The listing builds one solid part. Answer for the finished solid, in the listing's coordinates (mm). A direction names the side the tool comes from. Round coordinates to 2 decimals unless told otherwise and drop trailing zeros. Loops run counter-clockwise (first coordinate to the right, second up) from the corner with the lowest first, then second, coordinate; pieces in that order, holes last. Notation, with made-up numbers: (-25, 1.25) -> (12, 1.25) arc R23 ccw to (12, 30.25) -> close; hole circle Ø4 at (73, -31). An arc over 180 degrees is marked (long way). Use a Markdown table: item, result. Add a question column.
Q1. Section A-A on x = 0 is taken. Give the vertices of the cut face in (y, z).
Q2. Section B-B on z = -5 is taken. Give the vertices of the cut face in (x, y).
Q3. Which of the six approach directions +Z, -Z, +X, -X, +Y, -Y give full straight-line access (tool end or side, diameter ignored) to faces 1 (the flat face through (-1.4, 0, -4.5)), 2 (the cylindrical face through (-6, 31, 0))?
Q4. Consider line 1 (Y direction, x = -1.75, z = 5.5); line 2 (X direction, y = 19.5, z = 0.25); line 3 (X direction, y = 26.5, z = 2.5). Determine where each line is inside the solid, lowest interval first.
Q5. Section C-C on y = 22.5 is taken. Give the vertices of the cut face in (x, z), then the cut area to 3 significant figures.
Q6. Section D-D on z = 0 is taken. Give the vertices of the cut face in (x, y).
Q7. For a pull along Y with two mould halves and no side action, classify faces 3 (the cylindrical face through (-0.59, 14.79, -4.46)), 4 (the flat face through (0, -2, 0)), 5 (the cylindrical face through (-6, -1, 0)) as released by +Y, released by -Y, zero draft, split by the parting line, or undercut.
Q8. Given pin 1 Ø5 at (x, y) = (-4.5, 6.5) entering from +Z; pin 2 Ø1.5 at (y, z) = (26, 2) entering from -X; pin 3 Ø1 at (x, y) = (2, 2.5) entering from -Z, each flat-ended and moving along its own axis, determine where each tip first touches the part or whether it passes through.
from build123d import *

# Parameters (mm, degrees)
SKETCH1_R           = 4.5
BOSS_EXTRUDE1_DEPTH = 30
SKETCH2_R           = 6
BOSS_EXTRUDE2_DEPTH = 2
SKETCH3_R           = 6
BOSS_EXTRUDE3_DEPTH = 2


with BuildPart() as part:
    # Sketch1 → Boss-Extrude1 (new body)
    with BuildSketch(Plane(origin=(0, 0, 0), x_dir=(1, 0, 0), z_dir=(0, 1, 0))):
        Circle(SKETCH1_R)
    extrude(amount=BOSS_EXTRUDE1_DEPTH)

    # Sketch2 → Boss-Extrude2 (add)
    with BuildSketch(Plane(origin=(0, 0, 0), x_dir=(1, 0, 0), z_dir=(0, 1, 0))):
        Circle(SKETCH2_R)
    extrude(amount=-BOSS_EXTRUDE2_DEPTH)

    # Sketch3 → Boss-Extrude3 (add)
    with BuildSketch(Plane(origin=(0, 30, 0), x_dir=(1, 0, 0), z_dir=(0, 1, 0))):
        Circle(SKETCH3_R)
    extrude(amount=BOSS_EXTRUDE3_DEPTH)


solid = part.part
Checked values:
| question | item | result |
|---|---|---|
| 1 | outline | (-2, -6) -> (0, -6) -> (0, -4.5) -> (30, -4.5) -> (30, -6) -> (32, -6) -> (32, 6) -> (30, 6) -> (30, 4.5) -> (0, 4.5) -> (0, 6) -> (-2, 6) -> close |
| 2 | outline | (-3.32, -2) -> (3.32, -2) -> (3.32, 0) -> (-3.32, 0) -> close; (-3.32, 30) -> (3.32, 30) -> (3.32, 32) -> (-3.32, 32) -> close |
| 3 | face 1 | none |
| 3 | face 2 | +Y, -Y |
| 4 | line 1 | y = -2 to 0, 30 to 32 |
| 4 | line 2 | x = -4.49 to 4.49 |
| 4 | line 3 | x = -3.74 to 3.74 |
| 5 | outline | circle Ø9 at (0, 0) |
| 5 | area | 63.6 mm2 |
| 6 | outline | (-6, -2) -> (6, -2) -> (6, 0) -> (4.5, 0) -> (4.5, 30) -> (6, 30) -> (6, 32) -> (-6, 32) -> (-6, 30) -> (-4.5, 30) -> (-4.5, 0) -> (-6, 0) -> close |
| 7 | face 3 | undercut |
| 7 | face 4 | released by -Y |
| 7 | face 5 | zero draft |
| 8 | pin 1 | stops at z = 4.03 |
| 8 | pin 2 | stops at x = -4.32 |
| 8 | pin 3 | stops at z = -4.24 |
